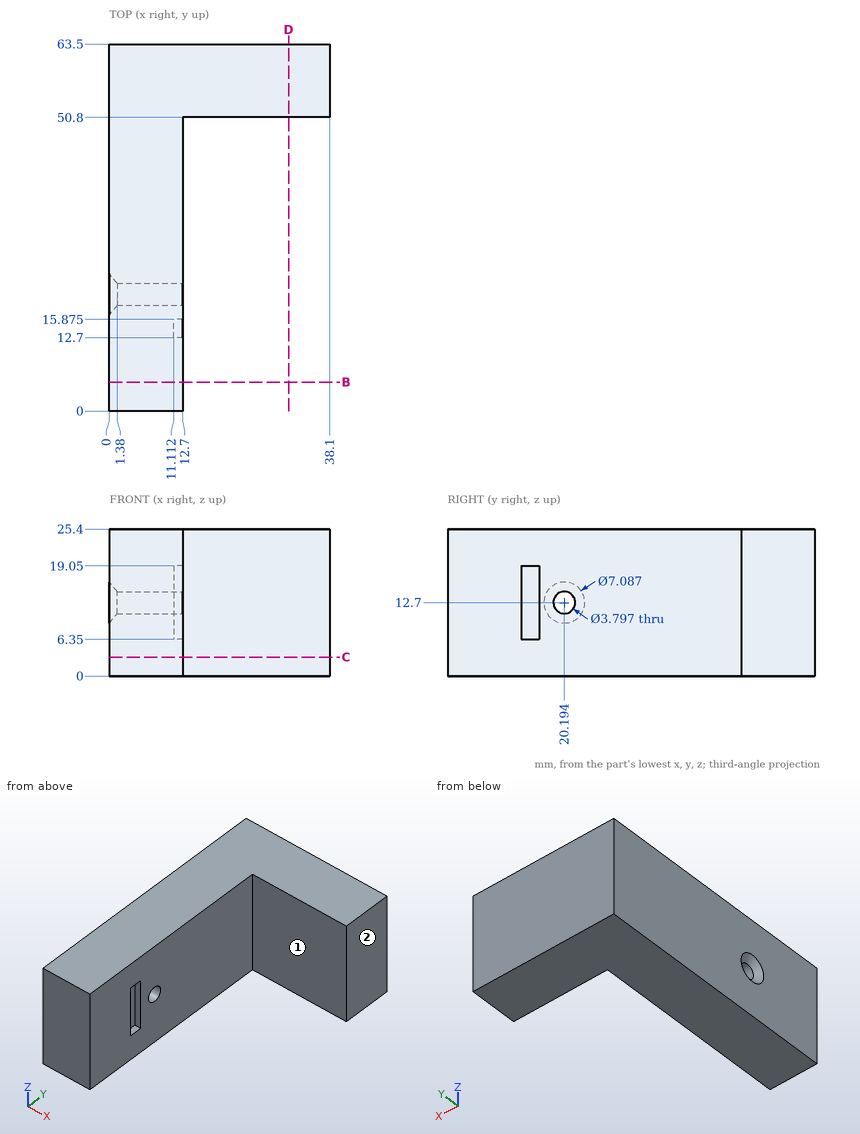
Print and shaded views of the part. All mm, measured from the part's lowest x, y and z. A direction names the side the tool comes from. Round coordinates to 2 decimals unless told otherwise and drop trailing zeros. Order: outer loops, then holes, each group sorted by start corner. A loop starts at its lowest first (then second) coordinate and runs counter-clockwise, first axis right, second up. Notation, with made-up numbers: (7, 88.5) - (23, 88.5) arc R35 ccw to (23, 127.5) - close; hole circle Ø1 at (88.5, -20). An arc over 180 degrees is marked (long way). Use a Markdown table: item, result.
1) Saw through at D-D on x = 31. Write the cut outline in (y, z), and give its area (3 significant figures).
Recorded:
| item | result |
|---|---|
| outline | (50.8, 0) - (63.5, 0) - (63.5, 25.4) - (50.8, 25.4) - close |
| area | 323 mm² |
2) Tool access for the marked faces 1 and 2: list every direction of +Z, -Z, +X, -X, +Y, -Y with a clear straight run to the whole face (end or side of a thin tool).
Recorded:
| item | result |
|---|---|
| face 1 | +Z, -Z, +X, -Y |
| face 2 | +Z, -Z, +X, +Y, -Y |
3) Wall check: L1, parallel to Y at x = 9.5, z = 12.7 (1 decimal); L2, parallel to X at y = 47, z = 7.75; L3, parallel to Z at x = 11.5, y = 20.5 (1 decimal). Give the ranges that are in metal, low to high.
Recorded:
| item | result |
|---|---|
| L1 | y = 0 to 18.3, 22.1 to 63.5 |
| L2 | x = 0 to 12.7 |
| L3 | z = 0 to 10.8, 14.6 to 25.4 |
4) Saw through at C-C on z = 3.25. Write the cut outline in (x, y), and give its area (3 significant figures).
Recorded:
| item | result |
|---|---|
| outline | (0, 0) - (12.7, 0) - (12.7, 50.8) - (38.1, 50.8) - (38.1, 63.5) - (0, 63.5) - close |
| area | 1,130 mm² |
5) Saw through at B-B on y = 5. Write the cut outline in (x, z).
Recorded:
| item | result |
|---|---|
| outline | (0, 0) - (12.7, 0) - (12.7, 25.4) - (0, 25.4) - close |
6) Flat gauge pins, fed straight in: pin 1 Ø4 at (x, z) = (33, 11.5) entering from -Y; pin 2 Ø4 at (x, y) = (4.5, 15) entering from -Z; pin 3 Ø7.5 at (y, z) = (31, 14) entering from +X. Where does each tip first touch, or does it go through?
Recorded:
| item | result |
|---|---|
| pin 1 | stops at y = 50.8 |
| pin 2 | stops at z = 0 |
| pin 3 | stops at x = 12.7 |
